Autodesk Inventor part; units mm, degrees
ref_plane "YZ Plane" through (0, 0, 0) normal (1, 0, 0) x (0, 1, 0)
ref_plane "XZ Plane" through (0, 0, 0) normal (0, 1, 0) x (-1, 0, 0)
ref_plane "XY Plane" through (0, 0, 0) normal (0, 0, 1) x (1, 0, 0)
sketch "Sketch1" plane through (0, 0, 0) normal (0, 0, 1) x (1, 0, 0)
  line L0 (-29, 10) -> (29, 10)
  line L1 (29, 10) -> (29, -10)
  line L2 (29, -10) -> (-29, -10)
  line L3 (-29, -10) -> (-29, 10)
  line L4 (-29, 10) -> (29, -10) construction
  line L5 (29, 10) -> (-29, -10) construction
  point P0 (0, 0)
  dimension "d0" = 58
  dimension "d1" = 20
extrude "Extrusion1" add sketch "Sketch1" along normal blind 15
sketch "Sketch3" plane through (0, 0, 0) normal (0, 0, 1) x (1, 0, 0)
  line L0 (-29, -10) -> (29, -10)
  line L1 (29, -10) -> (29, 10)
  line L2 (29, 10) -> (-29, 10)
  line L3 (-29, 10) -> (-29, -10)
  line L4 (-40.6, 0) -> (40.6, 0)
  line L5 (0, -12.225) -> (0, 13.85)
  circle A0 centre (18.95, 7.75) radius 4.125
  circle A1 centre (-18.95, 7.75) radius 4.125
  point P0 (0, 0)
  point P1 (-22.4073, 10)
  point P2 (-15.4927, 10)
  point P3 (15.4927, 10)
  point P4 (22.4073, 10)
  dimension "d4" = 8.25
  dimension "d5" = 8.25
  dimension "d6" = 37.9
  dimension "d7" = 2.25
extrude "Extrusion2" cut sketch "Sketch3" along normal through all contours L2 A1 | L2 A0 picked at (-19.324, 7.5879) picked at (18.8469, 7.6595)
sketch "Sketch4" plane through (-15.4927, 10, 0) normal (0, 1, 0) x (1, 0, 0)
  line L0 (0, 0) -> (0, -15)
  line L1 (30.9853, -15) -> (0, -15)
  line L2 (30.9853, -15) -> (30.9853, 0)
  line L3 (30.9853, 0) -> (0, 0)
  line L4 (-25.1073, 0) -> (56.0927, 0)
  line L5 (15.4927, 0) -> (15.4927, -15) construction
  line L6 (30.9853, -15) -> (0, -15) construction
  line L7 (30.9853, -15) -> (30.9853, 0) construction
  line L8 (30.9853, -7.5) -> (0, -7.5) construction
  line L9 (4.2927, -5.25) -> (26.6927, -5.25)
  line L10 (26.6927, -5.25) -> (26.6927, -9.75)
  line L11 (26.6927, -9.75) -> (4.2927, -9.75)
  line L12 (4.2927, -9.75) -> (4.2927, -5.25)
  line L13 (4.2927, -5.25) -> (26.6927, -9.75)
  line L14 (26.6927, -5.25) -> (4.2927, -9.75)
  point P0 (15.4927, -7.5)
  dimension "d12" = 22.4
  dimension "d13" = 4.5
sketch "Sketch5" plane through (0, 0, 0) normal (0, 1, 0) x (-1, 0, 0)
  line L0 (15.4927, 0) -> (15.4927, 15)
  line L1 (-15.4927, 15) -> (15.4927, 15)
  line L2 (-15.4927, 15) -> (-15.4927, 0)
  line L3 (-15.4927, 0) -> (15.4927, 0)
  line L4 (40.6, 0) -> (-40.6, 0)
  line L5 (0, -3.05) -> (0, 18.3)
  line L6 (11.25, 9.75) -> (-11.25, 9.75)
  line L7 (-11.25, 9.75) -> (-11.25, 15.25)
  line L8 (-11.25, 15.25) -> (11.25, 15.25)
  line L9 (11.25, 15.25) -> (11.25, 9.75)
  line L10 (11.25, 9.75) -> (-11.25, 15.25) construction
  line L11 (-11.25, 9.75) -> (11.25, 15.25) construction
  point P0 (0, 0)
  point P1 (0, 12.5)
  dimension "d10" = 22.5
  dimension "d11" = 5.5
extrude "Extrusion3" cut sketch "Sketch4" against normal blind 10 contours L13 L14 L12 | L9 L14 L13 | L10 L13 L14 | L14 L13 L11
sketch "Sketch6" plane through (0, 0, 0) normal (0, 0, -1) x (-1, 0, 0)
  line L0 (11.2, 0) -> (-11.2, 0)
  arc A0 (15.4927, 10) -> (22.4073, 10) centre (18.95, 7.75) ccw
  line L1 (-15.4927, 10) -> (15.4927, 10)
  arc A1 (-22.4073, 10) -> (-15.4927, 10) centre (-18.95, 7.75) ccw
  line L2 (-29, 10) -> (-22.4073, 10)
  line L3 (-29, -10) -> (-29, 10)
  line L4 (29, -10) -> (-29, -10)
  line L5 (29, 10) -> (29, -10)
  line L6 (22.4073, 10) -> (29, 10)
  line L7 (40.6, 0) -> (-40.6, 0)
  line L8 (0, -14.25) -> (0, 15.5)
  circle A2 centre (0, 7.75) radius 5.25
  point P0 (0, 0)
  dimension "d16" = 10.5
extrude "Extrusion4" cut sketch "Sketch6" against normal through all contours A2 L1 L8 | L8 L1 A2 | L8 A2 L1 | L1 A2 L8
sketch "Sketch8" plane through (0, 0, 15) normal (0, 0, 1) x (1, 0, 0)
  arc A0 (-4.7434, 10) -> (4.7434, 10) centre (0, 7.75) ccw
  line L0 (-4.7434, 10) -> (-15.4927, 10)
  arc A1 (-22.4073, 10) -> (-15.4927, 10) centre (-18.95, 7.75) ccw
  line L1 (-22.4073, 10) -> (-29, 10)
  line L2 (-29, 10) -> (-29, -10)
  line L3 (-29, -10) -> (29, -10)
  line L4 (29, -10) -> (29, 10)
  line L5 (29, 10) -> (22.4073, 10)
  arc A2 (15.4927, 10) -> (22.4073, 10) centre (18.95, 7.75) ccw
  line L6 (15.4927, 10) -> (4.7434, 10)
  line L7 (-40.6, 0) -> (40.6, 0)
  line L8 (0, -14) -> (0, 14)
  line L9 (-29, 10) -> (-29, -10)
  line L10 (29, -10) -> (-29, -10)
  line L11 (-29, -10) -> (-29, -1.25)
  line L12 (-29, -1.25) -> (29, -1.25)
  line L13 (29, -1.25) -> (29, -10)
  point P0 (0, 0)
  point P1 (29, -1.25)
  dimension "d19" = 9
extrude "Extrusion5" add sketch "Sketch8" along normal blind 34.3 contours L12 L4 L3 L8 | L8 L3 L2 L12
fillet "Fillet4" radius 1 4 edges at (-29, -5.625, 49.3) (29, -5.625, 49.3) (-29, 4.375, 15) (29, 4.375, 15)
fillet "Fillet5" radius 1 2 edges at (-29, 0, 0) (29, 0, 0)
fillet "Fillet6" radius 0.5 4 edges at (-11.2, 5, 5.25) (-11.2, 5, 9.75) (11.2, 5, 5.25) (11.2, 5, 9.75)
equation "\"BendRadius\" = Thickness"
equation "\"BendReliefWidth\" = Thickness"
equation "\"BendReliefDepth\" = 0.5 * Thickness"
equation "\"CornerReliefSize\" = 4 * Thickness"
equation "\"MinimumRemnant\" = 2 * Thickness"
equation "\"TransitionRadius\" = BendRadius"
equation "\"JacobiRadiusSize\" = BendRadius"
equation "\"GapSize\" = Thickness"
properties part number "_3DPrint"
For this review, take the finished solid that the model builds, in its own axes (mm). A direction names the side the tool comes from. Coordinates: 2 decimals unless noted, no trailing zeros. Loops run counter-clockwise (first coordinate to the right, second up) from the corner with the lowest first, then second, coordinate; pieces in that order, holes last. Notation, with made-up numbers: (74.5, -29) - (108.5, -29) arc R15 cw to (108.5, -4) - close; hole circle Ø10 at (-23, 36). An arc over 180 degrees is marked (long way). Use a Markdown table: item, result. Add a question column.
Item 1: We need section C-C (x = -6). Give the boundary of the cut face in (y, z).
Item 2: We need section D-D (z = 43.5). Give the boundary of the cut face in (x, y), and give its area (4 significant figures).
Item 3: We need section A-A (y = 7.75). Give the number of separate pieces and of enclosed holes in the cut face, and give its area (3 significant figures).
Item 4: Tool access review of faces 1 (the face through (11.2, 5, 7)), 2 (the face through (19.074, 3.627, 7.395)), 3 (the face through (0, 2, 15)): name each direction out of +Z, -Z, +X, -X, +Y, -Y from which nothing blocks a thin tool from reaching the whole face with its end or side.
Item 5: For line 1 (X direction, y = 7.75, z = 12.65) (3 decimals); line 2 (X direction, y = 7.75, z = 6) (3 decimals); line 3 (Z direction, x = -9, y = 3.5), list the stretches that pass through material, from the lowest coordinate up.
Item 6: Insertion check: pin 1 Ø1.3 at (x, z) = (-2, 7) entering from +Y; pin 2 Ø8 at (x, y) = (-3, 5) entering from +Z; pin 3 Ø5 at (x, y) = (10, -6) entering from -Z. Each pin has a flat end and moves straight along its axis. Give the tip position at first contact, or say it passes through.
Item 7: We need section B-B (y = 1.5). Give the boundary of the cut face in (x, z), and give its area (3 significant figures).
Item 8: Mouldability with a two-part tool opening along Y and no side actions: class faces 4 (the face through (0, -10, 24)), 5 (the face through (26, 10, 7)), 6 (the face through (-18.826, 3.627, 7.395)) as pulls with the +Y half, pulls with the -Y half, needs draft (parallel to the pull), parting line crosses it, or undercut.
Results list:
| question | item | result |
|---|---|---|
| 1 | outline | (-10, 0) - (10, 0) - (10, 5.25) - (0, 5.25) - (0, 9.75) - (10, 9.75) - (10, 15) - (-1.25, 15) - (-1.25, 49.3) - (-10, 49.3) - close |
| 2 | outline | (-29, -10) - (29, -10) - (29, -1.25) - (-29, -1.25) - close |
| 2 | area | 507.5 mm^2 |
| 3 | separate pieces | 4 |
| 3 | enclosed holes | 0 |
| 3 | area | 411 mm^2 |
| 4 | face 1 | +Y |
| 4 | face 2 | +Z, -Z |
| 4 | face 3 | +Z, +X, -X, +Y |
| 5 | line 1 | x = -29 to -23.075, -14.825 to -5.25, 5.25 to 14.825, 23.075 to 29 |
| 5 | line 2 | x = -29 to -23.075, -14.825 to -11.2, 11.2 to 14.825, 23.075 to 29 |
| 5 | line 3 | z = 0 to 5.25, 9.75 to 15 |
| 6 | pin 1 | stops at y = 0 |
| 6 | pin 2 | stops at z = 15 |
| 6 | pin 3 | stops at z = 0 |
| 7 | outline | (-29, 1) arc R1 ccw to (-28, 0) - (28, 0) arc R1 ccw to (29, 1) - (29, 14) arc R1 ccw to (28, 15) - (-28, 15) arc R1 ccw to (-29, 14) - close; hole (-11.2, 5.75) arc R0.5 ccw to (-10.7, 5.25) - (10.7, 5.25) arc R0.5 ccw to (11.2, 5.75) - (11.2, 9.25) arc R0.5 ccw to (10.7, 9.75) - (-10.7, 9.75) arc R0.5 ccw to (-11.2, 9.25) - close |
| 7 | area | 769 mm^2 |
| 8 | face 4 | pulls with the -Y half |
| 8 | face 5 | pulls with the +Y half |
| 8 | face 6 | undercut |
